Source: CAD feature listing. Evaluate the final solid. Frame: model axes, mm. Face numbers are marked on the shaded views. Round coordinates to 2 decimals unless told otherwise and drop trailing zeros. Write each loop counter-clockwise with the first axis right and the second up, starting at its lowest first coordinate (ties: lowest second). Pieces come first, ordered by that corner, then holes. Notation, with made-up numbers: (81.25, -20) - (135.25, -20) arc R16 cw to (135.25, -9) - close; hole circle Ø7 at (-13.5, 72.25). An arc over 180 degrees is marked (long way). Write item = value, one per line. Start each with the question number.
```python
from build123d import *

# Parameters (mm, degrees)
SKETCH_1_W          = 28
SKETCH_1_H          = 12
SKETCH_1_R          = 2
EXTRUDE_1_DEPTH     = 1.5
SKETCH_2_W          = 5
SKETCH_2_H          = 8
EXTRUDE_2_DEPTH     = 3
SKETCH_4_R          = 1.25
CUT_EXTRUDE_2_DEPTH = 5
FILLET_1_R          = 2
FILLET_2_R          = 1


with BuildPart() as part:
    # 草图1 → 凸台-拉伸1 (new, symmetric)
    with BuildSketch(Plane.XY):
        with Locations((0, 6)):
            Rectangle(SKETCH_1_W, SKETCH_1_H)
        with Locations((0, 3)):
            Circle(SKETCH_1_R, mode=Mode.SUBTRACT)
        with Locations(Location((0, 9, 0), (0, 0, 180))):
            Circle(SKETCH_1_R, mode=Mode.SUBTRACT)
    extrude(amount=EXTRUDE_1_DEPTH, both=True)

    # 草图2 → 凸台-拉伸2 (add)
    with BuildSketch(Plane.ZY.offset(14)):
        with Locations((4, 2)):
            Rectangle(SKETCH_2_W, SKETCH_2_H)
        with Locations((-4, 2)):
            Rectangle(SKETCH_2_W, SKETCH_2_H)
    extrude_2 = extrude(amount=-EXTRUDE_2_DEPTH)

    # 草图4 → 切除-拉伸2 (cut)
    with BuildSketch(Plane.ZY.offset(14)):
        with Locations((4, 2)):
            Circle(SKETCH_4_R)
        with Locations((-4, 2)):
            Circle(SKETCH_4_R)
    cut_extrude_2 = extrude(amount=-CUT_EXTRUDE_2_DEPTH, mode=Mode.SUBTRACT)

    # 镜向1: 凸台-拉伸2, 切除-拉伸2 across plane
    add(extrude_2.mirror(Plane(origin=(0, 0, 0), x_dir=(0, 0, 1), z_dir=(1, 0, 0))))
    add(cut_extrude_2.mirror(Plane(origin=(0, 0, 0), x_dir=(0, 0, 1), z_dir=(1, 0, 0))), mode=Mode.SUBTRACT)

    # 圆角1
    fillet_1_edges = [part.edges().sort_by_distance(p)[0] for p in [
        (-12.5, 6, 1.5),
        (-12.5, 6, 6.5),
        (-12.5, -2, 6.5),
        (-12.5, 6, -6.5),
        (-12.5, 6, -1.5),
        (-12.5, -2, -6.5),
        (12.5, 6, 1.5),
        (12.5, -2, 6.5),
        (12.5, 6, 6.5),
        (-14, 12, 0),
        (12.5, 6, -1.5),
        (14, 12, 0),
        (12.5, 6, -6.5),
        (12.5, -2, -6.5),
    ]]
    fillet(fillet_1_edges, radius=FILLET_1_R)

    # 圆角2
    fillet_2_edges = [part.edges().sort_by_distance(p)[0] for p in [
        (12.5, 0, -1.5),
        (12.5, 0, 1.5),
        (-12.5, 0, 1.5),
        (-12.5, 0, -1.5),
    ]]
    fillet(fillet_2_edges, radius=FILLET_2_R)
    fillet_2_2_edges = [part.edges().sort_by_distance(p)[0] for p in [
        (12.5, -2, -1.5),
        (12.5, -2, 1.5),
        (-12.5, -2, 1.5),
        (-12.5, -2, -1.5),
    ]]
    fillet(fillet_2_2_edges, radius=FILLET_2_R - 0.0001)  # a hair under: the kernel refuses the full size


solid = part.part
```
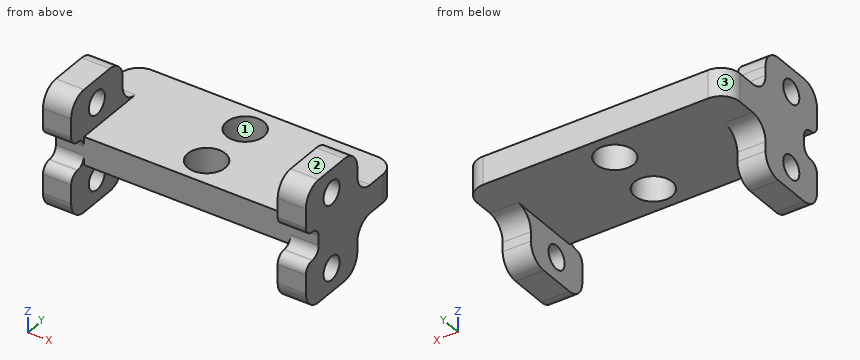
(1) Contact query for flat-ended pins moving along their axis: P1, Ø3.5, axis at x = 6.5, y = 3.5, coming from the -Z side; P2, Ø2.5, axis at x = 6.5, z = -0.5, coming from the -Y side; P3, Ø3.5, axis at x = 6, y = 5, coming from the +Z side. Output: stop coordinate, or through.
(2) Section C-C (z = 1). Return the cut outline in (x, y).
(3) Section A-A (x = 0). Return the cut outline in (y, z).
(4) Section D-D (x = -3). Return the cut outline in (y, z).
(5) Ray query, L1, parallel to Y at x = 0, z = -0.25; L2, parallel to Z at x = 12.7, y = 2; L3, parallel to Y at x = -12.9, z = -4. Return the intervals inside material, ascending. Write a range as from..to.
(6) Section B-B (y = 8.5). Return the cut outline in (x, z), plus the area to 3 significant figures.
(7) Pull-direction query (X, two-part tool) for the marked faces 1, 2 and 3; classes: +X half, -X half, draft (parallel to the pull), parting line (faces both ways), or undercut.
Solution:
q1.P1 = -1.5
q1.P2 = 0
q1.P3 = 1.5
q2.outline = (-14, -0.13) - (-11, -0.13) - (-11, 0) - (11, 0) - (11, -0.13) - (14, -0.13) - (14, 10) arc R2 ccw to (12, 12) - (-12, 12) arc R2 ccw to (-14, 10) - close; hole circle Ø4 at (0, 3); hole circle Ø4 at (0, 9)
q3.outline = (0, -1.5) - (1, -1.5) - (1, 1.5) - (0, 1.5) - close; (5, -1.5) - (7, -1.5) - (7, 1.5) - (5, 1.5) - close; (11, -1.5) - (12, -1.5) - (12, 1.5) - (11, 1.5) - close
q4.outline = (0, -1.5) - (12, -1.5) - (12, 1.5) - (0, 1.5) - close
q5.L1 = 0..1, 5..7, 11..12
q5.L2 = -6.5..-5.25, -2.75..2.75, 5.25..6.5
q5.L3 = -2..0.75, 3.25..6
q6.outline = (-14, -1.5) - (-1.94, -1.5) - (-1.94, 1.5) - (-14, 1.5) - close; (1.94, -1.5) - (14, -1.5) - (14, 1.5) - (1.94, 1.5) - close
q6.area = 72.4 mm^2
q7.face_1 = undercut
q7.face_2 = draft
q7.face_3 = -X half
